The listing builds one solid part. Answer for the finished solid, in the listing's coordinates (mm). A direction names the side the tool comes from. Round coordinates to 2 decimals unless told otherwise and drop trailing zeros. Write each loop counter-clockwise with the first axis right and the second up, starting at its lowest first coordinate (ties: lowest second). Pieces come first, ordered by that corner, then holes.
Item 1: Find section B-B on z = -252. Give the vertices of the cut face in (x, y) (3 decimals).
Item 2: Find section A-A on y = -8. Give the vertices of the cut face in (x, z) (3 decimals), then the cut area to 3 significant figures.
Item 3: Find the intervals of material crossed by probe 1 along X at (y, z) = (-15, 206) (3 decimals); probe 2 along X at (y, z) = (-23, 260); probe 3 along Y at (x, z) = (1.25, -259) (3 decimals), in increasing order.
Item 4: A tool of negligible diameter and unlimited length cuts with its end or side. For faces 1 (the face through (-12.7, 0, 5)), 2 (the face through (9.525, 0, 5)), from which of +Z, -Z, +X, -X, +Y, -Y can it reach the whole face along a straight path? Write none if from no direction.
Item 5: For a pull along Y with two mould halves and no side action, classify faces 3 (the face through (0, -22.225, 5)), 4 (the face through (-10, -2, 323.85)), 5 (the face through (0, 25.4, 5)) as +Y half, -Y half, draft (parallel to the pull), parting line (faces both ways), or undercut.
```python
from build123d import *

# Parameters (mm, degrees)
SKETCH1_W           = 25.4
SKETCH1_H           = 50.8
SKETCH1_W_2         = 19.05
SKETCH1_H_2         = 44.45
BOSS_EXTRUDE1_DEPTH = 323.85
CUT_EXTRUDE1_REACH  = 330.056
SKETCH2_R           = 2.1971


with BuildPart() as part:
    # Sketch1 → Boss-Extrude1 (new, symmetric)
    with BuildSketch(Plane.XY):
        Rectangle(SKETCH1_W, SKETCH1_H)
        Rectangle(SKETCH1_W_2, SKETCH1_H_2, mode=Mode.SUBTRACT)
    extrude(amount=BOSS_EXTRUDE1_DEPTH, both=True)

    # Cut-Extrude1: up to this face of the body (flat: up to its plane)
    cut_extrude1_end = Plane(part.part.faces().sort_by_distance((0, -25.4, 0))[0])
    # Sketch2 → Cut-Extrude1 (cut, up to the picked face)
    with BuildSketch(Plane(origin=(0, 25.4, 0), x_dir=(1, 0, 0), z_dir=(0, 1, 0)), mode=Mode.PRIVATE) as cut_extrude1_sk1:
        with Locations(Location((8.2464e-05, -304.8, 0), (0, 0, 270))):
            Circle(SKETCH2_R)
    cut_extrude1_tool1 = split(extrude(cut_extrude1_sk1.sketch, amount=-CUT_EXTRUDE1_REACH, mode=Mode.PRIVATE), bisect_by=cut_extrude1_end, keep=Keep.BOTH, mode=Mode.PRIVATE)
    # Sketch2 → Cut-Extrude1 (cut, up to the picked face)
    with BuildSketch(Plane(origin=(0, 25.4, 0), x_dir=(1, 0, 0), z_dir=(0, 1, 0)), mode=Mode.PRIVATE) as cut_extrude1_sk2:
        with Locations(Location((8.2464e-05, -260.35, 0), (0, 0, 270))):
            Circle(SKETCH2_R)
    cut_extrude1_tool2 = split(extrude(cut_extrude1_sk2.sketch, amount=-CUT_EXTRUDE1_REACH, mode=Mode.PRIVATE), bisect_by=cut_extrude1_end, keep=Keep.BOTH, mode=Mode.PRIVATE)
    # Sketch2 → Cut-Extrude1 (cut, up to the picked face)
    with BuildSketch(Plane(origin=(0, 25.4, 0), x_dir=(1, 0, 0), z_dir=(0, 1, 0)), mode=Mode.PRIVATE) as cut_extrude1_sk3:
        with Locations(Location((8.2464e-05, -171.45, 0), (0, 0, 270))):
            Circle(SKETCH2_R)
    cut_extrude1_tool3 = split(extrude(cut_extrude1_sk3.sketch, amount=-CUT_EXTRUDE1_REACH, mode=Mode.PRIVATE), bisect_by=cut_extrude1_end, keep=Keep.BOTH, mode=Mode.PRIVATE)
    add(cut_extrude1_tool1.solids().sort_by(Axis((8.2e-05, 25.4, 304.8), (0, -1, 0)))[0], mode=Mode.SUBTRACT)
    add(cut_extrude1_tool2.solids().sort_by(Axis((8.2e-05, 25.4, 260.35), (0, -1, 0)))[0], mode=Mode.SUBTRACT)
    add(cut_extrude1_tool3.solids().sort_by(Axis((8.2e-05, 25.4, 171.45), (0, -1, 0)))[0], mode=Mode.SUBTRACT)


solid = part.part
```
Check values:
1. outline: (-12.7, -25.4) - (12.7, -25.4) - (12.7, 25.4) - (-12.7, 25.4) - close; hole (-9.525, -22.225) - (9.525, -22.225) - (9.525, 22.225) - (-9.525, 22.225) - close
2. outline: (-12.7, -323.85) - (-9.525, -323.85) - (-9.525, 323.85) - (-12.7, 323.85) - close; (9.525, -323.85) - (12.7, -323.85) - (12.7, 323.85) - (9.525, 323.85) - close
2. area: 4,110 mm2
3. probe 1: x = -12.7 to -9.525, 9.525 to 12.7
3. probe 2: x = -12.7 to -2.17, 2.17 to 12.7
3. probe 3: y = -25.4 to -22.225, 22.225 to 25.4
4. face 1: +Z, -Z, -X, +Y, -Y
4. face 2: +Z, -Z
5. face 3: undercut
5. face 4: draft
5. face 5: +Y half
